Input: part model. Units: mm. Frame: model coordinates. A direction names the side the tool comes from. Give positions to 0.01 mm unless a question says otherwise; leave off trailing zeros. Loops run counter-clockwise (first coordinate to the right, second up) from the corner with the lowest first, then second, coordinate; pieces in that order, holes last.
from build123d import *

# Parameters (mm, degrees)
SKETCH1_R                = 34
BOSS_EXTRUDE1_DEPTH      = 10
SKETCH2_R                = 19.7871926
SKETCH2_R_2              = 2
CUT_EXTRUDE1_DEPTH       = 10
SKETCH3_R                = 4.837531333
SKETCH4_W                = 4.837531333
SKETCH4_H                = 4.837531333
CUT_EXTRUDE3_DEPTH       = 38
CUT_EXTRUDE3_DEPTH_BACK  = 38
SKETCH5_W                = 72.361656805
SKETCH5_H                = 8.896778435
BOSS_EXTRUDE2_START      = 60
SKETCH6_R                = 22.2871926
SKETCH6_R_2              = 19.7871926
BOSS_EXTRUDE2_DEPTH      = 60
SKETCH7_R                = 21.0371926
SKETCH7_R_2              = 19.7871926
CUT_EXTRUDE4_DEPTH       = 25
CUT_EXTRUDE6_DEPTH       = 25
CUT_EXTRUDE6_DEPTH_BACK  = 25
SKETCH8_R                = 2
CUT_EXTRUDE7_DEPTH       = 43
CUT_EXTRUDE7_DEPTH_BACK  = 53
SKETCH9_W                = 69.351432881
SKETCH9_H                = 5.737807944
CUT_EXTRUDE8_START       = -25
SKETCH10_R               = 22.2871926
SKETCH10_R_2             = 21.0371926
CUT_EXTRUDE8_DEPTH       = 25
CUT_EXTRUDE9_DEPTH       = 30
CUT_EXTRUDE9_DEPTH_BACK  = 30
SKETCH11_R               = 2
CUT_EXTRUDE10_DEPTH      = 53
CUT_EXTRUDE10_DEPTH_BACK = 26
SKETCH12_W               = 42.0743852
SKETCH12_H               = 25


with BuildPart() as part:
    # Sketch1 → Boss-Extrude1 (new body)
    with BuildSketch(Plane(origin=(0, 0, 0), x_dir=(1, 0, 0), z_dir=(0, 1, 0))):
        with Locations(Location((0, 0, 0), (0, 0, 270))):
            Circle(SKETCH1_R)
    extrude(amount=BOSS_EXTRUDE1_DEPTH)

    # Sketch2 → Cut-Extrude1 (cut)
    with BuildSketch(Plane.XZ):
        with Locations(Location((0, 0, 0), (0, 0, 270))):
            Circle(SKETCH2_R)
        with Locations(Location((-22.1, 12.5, 0), (0, 0, 270))):
            Circle(SKETCH2_R_2)
        with Locations(Location((22.1, 12.5, 0), (0, 0, 90))):
            Circle(SKETCH2_R_2)
        with Locations(Location((22.1, -12.5, 0), (0, 0, 270))):
            Circle(SKETCH2_R_2)
        with Locations(Location((-22.1, -12.5, 0), (0, 0, 90))):
            Circle(SKETCH2_R_2)
    extrude(amount=-CUT_EXTRUDE1_DEPTH, mode=Mode.SUBTRACT)

    # Sketch3 → Cut-Revolve1 (revolve, cut)
    with BuildSketch(Plane(origin=(0, 0, 0), x_dir=(0, 0, -1), z_dir=(1, 0, 0)), mode=Mode.PRIVATE) as cut_revolve1_sk:
        with Locations((-34, 5)):
            Circle(SKETCH3_R)
    revolve(cut_revolve1_sk.sketch.rotate(Axis((0, 0, 0), (0, 1, 0)), 180), axis=Axis((0, 0, 0), (0, 1, 0)), mode=Mode.SUBTRACT)

    # Sketch4 → Cut-Revolve2 (revolve, cut)
    with BuildSketch(Plane(origin=(0, 0, 0), x_dir=(0, 0, -1), z_dir=(1, 0, 0)), mode=Mode.PRIVATE) as cut_revolve2_sk:
        with Locations((-31.581234333, 2.581234333)):
            Rectangle(SKETCH4_W, SKETCH4_H)
    revolve(cut_revolve2_sk.sketch.rotate(Axis((0, 0, 0), (0, 1, 0)), 180), axis=Axis((0, 0, 0), (0, 1, 0)), mode=Mode.SUBTRACT)

    # Sketch5 → Cut-Extrude3 (cut, two sides: drawn at the far end of the back side and taken through both)
    with BuildSketch(Plane(origin=(0, 0, 0), x_dir=(0, 0, -1), z_dir=(1, 0, 0)).offset(-CUT_EXTRUDE3_DEPTH_BACK)):
        with Locations((-0.901301775, 0.551610782)):
            Rectangle(SKETCH5_W, SKETCH5_H)
    extrude(amount=CUT_EXTRUDE3_DEPTH + CUT_EXTRUDE3_DEPTH_BACK, mode=Mode.SUBTRACT)

    # Sketch6 → Boss-Extrude2 (add)
    with BuildSketch(Plane.XZ.offset(-5).offset(BOSS_EXTRUDE2_START)):
        with Locations(Location((0, 0, 0), (0, 0, 270))):
            Circle(SKETCH6_R)
        with Locations(Location((0, 0, 0), (0, 0, 270))):
            Circle(SKETCH6_R_2, mode=Mode.SUBTRACT)
    extrude(amount=-BOSS_EXTRUDE2_DEPTH)

    # Sketch7 → Cut-Extrude4 (cut)
    with BuildSketch(Plane.XZ.offset(55)):
        with Locations(Location((0, 0, 0), (0, 0, 270))):
            Circle(SKETCH7_R)
        with Locations(Location((0, 0, 0), (0, 0, 270))):
            Circle(SKETCH7_R_2, mode=Mode.SUBTRACT)
    extrude(amount=-CUT_EXTRUDE4_DEPTH, mode=Mode.SUBTRACT)

    # Sketch8 → Cut-Extrude6 (cut, two sides: drawn at the far end of the back side and taken through both)
    with BuildSketch(Plane(origin=(0, 0, 0), x_dir=(0, 0, -1), z_dir=(1, 0, 0)).offset(-CUT_EXTRUDE6_DEPTH_BACK)):
        with Locations(Location((0, -42.5, 0), (0, 0, 180))):
            Circle(SKETCH8_R)
    extrude(amount=CUT_EXTRUDE6_DEPTH + CUT_EXTRUDE6_DEPTH_BACK, mode=Mode.SUBTRACT)

    # Sketch9 → Cut-Extrude7 (cut, two sides: drawn at the far end of the back side and taken through both)
    with BuildSketch(Plane(origin=(0, 0, 0), x_dir=(0, 0, -1), z_dir=(1, 0, 0)).offset(-CUT_EXTRUDE7_DEPTH_BACK)):
        with Locations((0.165912519, 7.868903972)):
            Rectangle(SKETCH9_W, SKETCH9_H)
    extrude(amount=CUT_EXTRUDE7_DEPTH + CUT_EXTRUDE7_DEPTH_BACK, mode=Mode.SUBTRACT)

    # Sketch10 → Cut-Extrude8 (cut)
    with BuildSketch(Plane(origin=(0, 5, 0), x_dir=(1, 0, 0), z_dir=(0, 1, 0)).offset(CUT_EXTRUDE8_START)):
        with Locations(Location((0, 0, 0), (0, 0, 270))):
            Circle(SKETCH10_R)
        with Locations(Location((0, 0, 0), (0, 0, 90))):
            Circle(SKETCH10_R_2, mode=Mode.SUBTRACT)
    extrude(amount=CUT_EXTRUDE8_DEPTH, mode=Mode.SUBTRACT)

    # Sketch11 → Cut-Extrude9 (cut, two sides: drawn at the far end of the back side and taken through both)
    with BuildSketch(Plane(origin=(0, 0, 0), x_dir=(0, 0, -1), z_dir=(1, 0, 0)).offset(-CUT_EXTRUDE9_DEPTH_BACK)):
        with Locations(Location((0, -7.5, 0), (0, 0, 180))):
            Circle(SKETCH11_R)
    extrude(amount=CUT_EXTRUDE9_DEPTH + CUT_EXTRUDE9_DEPTH_BACK, mode=Mode.SUBTRACT)

    # Sketch12 → Cut-Extrude10 (cut, two sides: drawn at the far end of the back side and taken through both)
    with BuildSketch(Plane.XY.offset(-CUT_EXTRUDE10_DEPTH_BACK)):
        with Locations((0, -7.5)):
            Rectangle(SKETCH12_W, SKETCH12_H)
    extrude(amount=CUT_EXTRUDE10_DEPTH + CUT_EXTRUDE10_DEPTH_BACK, mode=Mode.SUBTRACT)


solid = part.part
(1) Reachability of faces 1 (the cylindrical face through (5.944, -25.07, -18.873)), 2 (the cylindrical face through (-20.537, -42.675, 4.56)) from +Z, -Z, +X, -X, +Y, -Y: full face, straight path, thin tool, end or side. Return the list, or none.
Values follow:
face 1: +Y, -Y
face 2: -Y
(2) Cut plane D-D (y = -39.5). Return the cut outline in (x, z), and give its area (3 significant figures).
Values follow:
outline: circle Ø44.57 at (0, 0); hole circle Ø42.07 at (0, 0)
area: 170 mm2
(3) Cut plane C-C (z = 5). Return the cut outline in (x, y), and give its area (3 significant figures).
Values follow:
outline: (-21.72, -55) - (-20.43, -55) - (-20.43, -30) - (-19.15, -30) - (-19.15, -20) - (-21.72, -20) - close; (19.15, -30) - (20.43, -30) - (20.43, -55) - (21.72, -55) - (21.72, -20) - (19.15, -20) - close
area: 116 mm2
(4) Mould query, pull axis X, two halves, no side actions, for faces 3 (the flat face through (20, -20, 0)), 4 (the cylindrical face through (22.098, -37.745, 2.901)), 5 (the flat face through (-19, -30, -8)). Classes: +X half, -X half, draft (parallel to the pull), parting line (faces both ways), or undercut.
Values follow:
face 3: draft
face 4: parting line
face 5: undercut
(5) Cut plane B-B (z = 0). Return the cut outline in (x, y).
Values follow:
outline: (-22.29, -55) - (-21.04, -55) - (-21.04, -44.5) - (-22.29, -44.5) - close; (-22.29, -40.5) - (-21.04, -40.5) - (-21.04, -30) - (-19.79, -30) - (-19.79, -20) - (-22.29, -20) - close; (19.79, -30) - (21.04, -30) - (21.04, -40.5) - (22.29, -40.5) - (22.29, -20) - (19.79, -20) - close; (21.04, -55) - (22.29, -55) - (22.29, -44.5) - (21.04, -44.5) - close
(6) Cut plane A-A (x = 0). Return the cut outline in (y, z).
Values follow:
outline: (-55, -22.29) - (-20, -22.29) - (-20, -19.79) - (-30, -19.79) - (-30, -21.04) - (-55, -21.04) - close; (-55, 21.04) - (-30, 21.04) - (-30, 19.79) - (-20, 19.79) - (-20, 22.29) - (-55, 22.29) - close
(7) Pin query (flat end, axial travel): pin 1 Ø3 at (y, z) = (-27, -11.5) entering from -X; pin 2 Ø12 at (y, z) = (-27.5, 7.5) entering from +X; pin 3 Ø10 at (y, z) = (-27, 9) entering from -X; pin 4 Ø1.5 at (x, z) = (16.5, -17.5) entering from +Y. Return the tip coordinate at first contact, or that it passes through.
Values follow:
pin 1: stops at x = -19.92
pin 2: stops at x = 22.24
pin 3: stops at x = -21.93
pin 4: passes through
(8) Ray query, probe 1 along X at (y, z) = (-22, 0); probe 2 along X at (y, z) = (-39.75, 0); probe 3 along Y at (x, z) = (21.7, 0). Return the intervals inside material, ascending.
Values follow:
probe 1: x = -22.29 to -19.79, 19.79 to 22.29
probe 2: x = -22.29 to -21.04, 21.04 to 22.29
probe 3: y = -55 to -44.5, -40.5 to -20
